```python
from build123d import *

# Parameters (mm, degrees)
BOSS_EXTRUDE1_DEPTH = 19
SKETCH2_R           = 8
CUT_EXTRUDE1_DEPTH  = 4
SKETCH3_R           = 3.3
CUT_EXTRUDE2_DEPTH  = 14
CHAMFER1_SIZE       = 2


with BuildPart() as part:
    # Sketch1 → Boss-Extrude1 (new body)
    with BuildSketch(Plane(origin=(0, 0, 0), x_dir=(1, 0, 0), z_dir=(0, 1, 0))):
        Polygon((0, 9), (-4.5, 7.794228634), (-7.794228634, 4.5), (-9, 0), (-7.794228634, -4.5), (-4.5, -7.794228634), (0, -9), (4.5, -7.794228634), (7.794228634, -4.5), (9, 0), (7.794228634, 4.5), (4.5, 7.794228634), align=None)
    extrude(amount=BOSS_EXTRUDE1_DEPTH)

    # Sketch2 → Cut-Extrude1 (cut)
    with BuildSketch(Plane(origin=(0, 19, 0), x_dir=(1, 0, 0), z_dir=(0, 1, 0))):
        Circle(SKETCH2_R)
    extrude(amount=-CUT_EXTRUDE1_DEPTH, mode=Mode.SUBTRACT)

    # Sketch3 → Cut-Extrude2 (cut)
    with BuildSketch(Plane(origin=(0, 15, 0), x_dir=(1, 0, 0), z_dir=(0, 1, 0))):
        Circle(SKETCH3_R)
    extrude(amount=-CUT_EXTRUDE2_DEPTH, mode=Mode.SUBTRACT)

    # Chamfer1
    chamfer1_edges = [part.edges().sort_by_distance(p)[0] for p in [
        (6.147114317, 0, -6.147114317),
        (8.397114317, 0, -2.25),
        (8.397114317, 0, 2.25),
        (6.147114317, 0, 6.147114317),
        (2.25, 0, 8.397114317),
        (-2.25, 0, 8.397114317),
        (-6.147114317, 0, 6.147114317),
        (-8.397114317, 0, 2.25),
        (-8.397114317, 0, -2.25),
        (-6.147114317, 0, -6.147114317),
        (-2.25, 0, -8.397114317),
        (2.25, 0, -8.397114317),
    ]]
    chamfer(chamfer1_edges, length=CHAMFER1_SIZE)


solid = part.part
```
CAD build for the part. Positions are in the model's coordinates, mm. Round coordinates to 2 decimals unless told otherwise and drop trailing zeros. Order: outer loops, then holes, each group sorted by start corner. A loop starts at its lowest first (then second) coordinate and runs counter-clockwise, first axis right, second up.
Item 1: Saw through at D-D on x = -1.25. Write the cut outline in (y, z), then the cut area to 3 significant figures.
Item 2: Saw through at C-C on x = -3.75. Write the cut outline in (y, z).
Item 3: Pin check, flat tips, straight feed: pin 1 (6 mm diameter, centred on x = 4, z = 1.5, fed in from +Y); pin 2 (1 mm diameter, centred on y = 15, z = 1.5, fed in from +X); pin 3 (2 mm diameter, centred on x = 4, y = 3, fed in from +Z). Stop position of each tip, or through.
Item 4: Probe line 1 along Z through (x, y) = (0, 9); line 2 along Z through (x, y) = (0, 16.6). List the from-to ranges inside material, lowest first.
Item 5: Saw through at B-B on z = 6.5. Write the cut outline in (x, y), then the cut area to 3 significant figures.
Item 6: Saw through at A-A on y = 6. Write the cut outline in (x, z).
Item 7: Mould opens along X. For faces 1 (the face through (-1.73, 17.03, 7.81)), 2 (the face through (-5, 19, -7)), 3 (the face through (2.219, 10.381, 8.406)), 4 (the face through (-5.407, 0.986, -5.453)) say: pulls with the +X half, pulls with the -X half, needs draft (parallel to the pull), parting line crosses it, or undercut.
Reported:
1. outline: (0, -6.59) - (2, -8.67) - (19, -8.67) - (19, -7.9) - (15, -7.9) - (15, -3.05) - (1, -3.05) - (1, 3.05) - (15, 3.05) - (15, 7.9) - (19, 7.9) - (19, 8.67) - (2, 8.67) - (0, 6.59) - close
1. area: 176 mm2
2. outline: (0, -5.72) - (0.55, -6.5) - (2, -8) - (19, -8) - (19, -7.07) - (15, -7.07) - (15, 7.07) - (19, 7.07) - (19, 8) - (2, 8) - (0.55, 6.5) - (0, 5.72) - close
3. pin 1: stops at y = 15
3. pin 2: stops at x = 8.73
3. pin 3: stops at z = 8.2
4. line 1: z = -9 to -3.3, 3.3 to 9
4. line 2: z = -9 to -8, 8 to 9
5. outline: (-5.79, 2) - (-3.75, 0.56) - (-1.6, 0) - (1.6, 0) - (3.75, 0.56) - (5.79, 2) - (5.79, 19) - (4.66, 19) - (4.66, 15) - (-4.66, 15) - (-4.66, 19) - (-5.79, 19) - close
5. area: 176 mm2
6. outline: (-9, 0) - (-7.79, -4.5) - (-4.5, -7.79) - (0, -9) - (4.5, -7.79) - (7.79, -4.5) - (9, 0) - (7.79, 4.5) - (4.5, 7.79) - (0, 9) - (-4.5, 7.79) - (-7.79, 4.5) - close; hole circle Ø6.6 at (0, 0)
7. face 1: undercut
7. face 2: needs draft
7. face 3: pulls with the +X half
7. face 4: pulls with the -X half
